from build123d import *

# Parameters (mm, degrees)
F0_W     = 226.934583
F0_H     = 125.4125
F0_R     = 2.15265
F0_R_2   = 9.525
F0_R_3   = 1.7272
F0_R_4   = 12.7
F1_DEPTH = 3.175
F2_R     = 23.8125


with BuildPart() as f1:
    # F0 (on Top) → F1 (new body)
    with BuildSketch(Plane.XY):
        with Locations((-113.467292, -62.70625)):
            Rectangle(F0_W, F0_H)
        with Locations((-212.647083, -120.015)):
            Circle(F0_R, mode=Mode.SUBTRACT)
        with Locations((-14.2875, -120.015)):
            Circle(F0_R, mode=Mode.SUBTRACT)
        with Locations((-106.960737, -59.198979)):
            Circle(F0_R, mode=Mode.SUBTRACT)
        with Locations((-95.735416, -47.973659)):
            Circle(F0_R_2, mode=Mode.SUBTRACT)
        with Locations((-84.510096, -59.198979)):
            Circle(F0_R, mode=Mode.SUBTRACT)
        with Locations((-106.960737, -36.748339)):
            Circle(F0_R, mode=Mode.SUBTRACT)
        with Locations((-84.510096, -36.748339)):
            Circle(F0_R, mode=Mode.SUBTRACT)
        with Locations((-37.282884, -37.282884)):
            Circle(F0_R_3, mode=Mode.SUBTRACT)
        with Locations((-10.342116, -37.282884)):
            Circle(F0_R_3, mode=Mode.SUBTRACT)
        with Locations((-23.8125, -23.8125)):
            Circle(F0_R_4, mode=Mode.SUBTRACT)
        with Locations((-37.282884, -10.342116)):
            Circle(F0_R_3, mode=Mode.SUBTRACT)
        with Locations((-10.342116, -10.342116)):
            Circle(F0_R_3, mode=Mode.SUBTRACT)
    extrude(amount=F1_DEPTH)

    # F2
    f2_edges = [f1.edges().sort_by_distance(p)[0] for p in [
        (0, 0, 1.5875),
    ]]
    fillet(f2_edges, radius=F2_R)


solid = f1.part
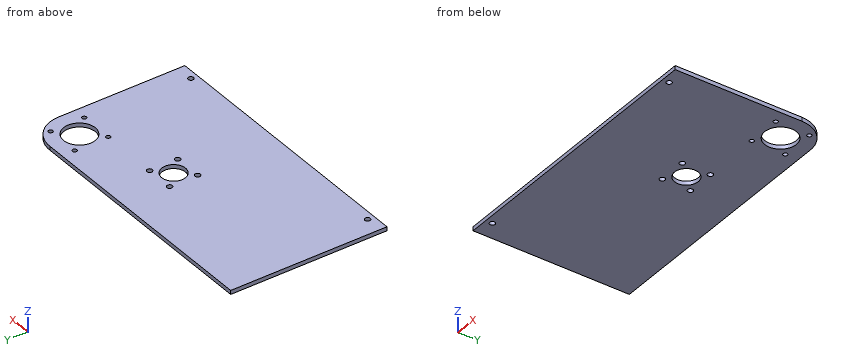
Design review of the part built by this model. Coordinates are the model's own, in mm. Give positions to 0.01 mm unless a question says otherwise; leave off trailing zeros. Loops run counter-clockwise (first coordinate to the right, second up) from the corner with the lowest first, then second, coordinate; pieces in that order, holes last. Notation, with made-up numbers: (-28, 21.25) - (20, 21.25) arc R18 ccw to (20, 36.25) - close; hole circle Ø8 at (42.25, -19). An arc over 180 degrees is marked (long way). Write item = value, one per line.
1) Take a section at A-A on y = -21. State the section outline as (x, z) points (3 decimals), and give its area (3 significant figures).
Result sheet:
outline = (-226.935, 0) - (-36.197, 0) - (-36.197, 3.175) - (-226.935, 3.175) - close; (-11.428, 0) - (-0.167, 0) - (-0.167, 3.175) - (-11.428, 3.175) - close
area = 641 mm2
2) To check wall thickness, follow line 1 (X direction, y = -37, z = 1.3); line 2 (X direction, y = -119, z = 2.9); line 3 (Y direction, x = -96, z = 1.95). State the ranges of each line that lie inside material, in increasing order.
Result sheet:
line_1 = -226.93 to -109.1, -104.82 to -86.65, -82.37 to -38.99, -35.58 to -12.05, -8.64 to 0
line_2 = -226.93 to -214.55, -210.75 to -16.19, -12.39 to 0
line_3 = -125.41 to -57.49, -38.45 to 0
3) Take a section at B-B on z = 1.35. Count the separate pieces of the cut face and the enclosed holes in it, and give its area (3 significant figures).
Result sheet:
separate_pieces = 1
enclosed_holes = 12
area = 27,400 mm2
4) Take a section at C-C on y = -54.5. State the section outline as (x, z) points (3 decimals), and give its area (3 significant figures).
Result sheet:
outline = (-226.935, 0) - (-102.673, 0) - (-102.673, 3.175) - (-226.935, 3.175) - close; (-88.798, 0) - (0, 0) - (0, 3.175) - (-88.798, 3.175) - close
area = 676 mm2
5) Clearance check with a flat-ended pin moving along its axis: pin 1 Ø4 at (x, y) = (-37.28, -37.28) entering from -Z. State where the tip first meets the part, or that it passes through.
Result sheet:
pin_1 = 0
